```python
from build123d import *

# Parameters (mm, degrees)
F0_R     = 4
F0_R_2   = 5
F1_DEPTH = 10


with BuildPart() as f1:
    # F0 (on Front) → F1 (new body)
    with BuildSketch(Plane.XZ):
        with BuildLine():
            ThreePointArc((-128.8754135109, -25.0952865806), (-123.1602737314, -22.4552566283), (-120.8289454463, -16.6073946878))
            ThreePointArc((-120.8289454463, -16.6073946878), (-124.0394968392, -9.9536939557), (-131.2458239011, -8.326357495))
            ThreePointArc((-131.2458239011, -8.326357495), (-137.7452743032, -17.797104136), (-128.8754135109, -25.0952865806))
        make_face()
        with Locations((-129.3289454463, -16.6073946878)):
            Circle(F0_R, mode=Mode.SUBTRACT)
        with BuildLine():
            ThreePointArc((-131.2458239011, -8.326357495), (-124.0394968392, -9.9536939557), (-120.8289454463, -16.6073946878))
            ThreePointArc((-120.8289454463, -16.6073946878), (-123.1602737314, -22.4552566283), (-128.8754135109, -25.0952865806))
            add(Edge.make_bspline(
                [(27.532273017, -23.963665398), (1.5839289913, -22.6401279773), (-50.8745236246, -19.0093143919), (-102.6400941915, -24.2784335073), (-128.8754135109, -25.0952865806)],
                knots=[0.0136350591, 0.0136350591, 0.0136350591, 0.0136350591, 0.501767797, 1, 1, 1, 1], degree=3))
            ThreePointArc((27.532273017, -23.963665398), (23.6774268876, -21.8978591269), (21.6302831699, -18.0330697627))
            add(Edge.make_bspline(
                [(21.6302831699, -18.0330697627), (10.6563367579, -17.139313249), (-11.4221872367, -15.3394334373), (-44.3388932106, -14.1423054761), (-78.9588463965, -16.6641001427), (-98.3406285912, -18.1155278421)],
                knots=[0, 0, 0, 0, 0.2993707154, 0.6024154943, 0.9795111889, 0.9795111889, 0.9795111889, 0.9795111889], degree=3))
            ThreePointArc((-98.3406285912, -18.1155278421), (-100.8823299041, -17.4386421951), (-102.4541582861, -15.3296672591))
            Line((-102.4541582861, -15.3296672591), (-104.3954498587, -9.1735058104))
            ThreePointArc((-104.3954498587, -9.1735058104), (-104.0739536016, -6.0220282679), (-101.5614502719, -4.0926507615))
            add(Edge.make_bspline(
                [(83.1727162004, 25.6010051817), (69.0016849645, 24.6252928547), (38.5314258984, 22.5273363348), (-18.4508975965, 16.7813390569), (-72.1336091939, 3.3504452865), (-101.5614502719, -4.0926507615)],
                knots=[0, 0, 0, 0, 0.2783902325, 0.5985889357, 0.9821534138, 0.9821534138, 0.9821534138, 0.9821534138], degree=3))
            add(Edge.make_bspline(
                [(83.1727162004, 25.6010051817), (75.1220807527, 20.7720126759), (58.4321749927, 10.7605519796), (43.1575612073, -4.5557382523), (35.2562556315, -12.4808577154)],
                knots=[0, 0, 0, 0, 0.4823562569, 1, 1, 1, 1], degree=3))
            ThreePointArc((35.2562556315, -12.4808577154), (36.1775577554, -14.4533773309), (36.4935331712, -16.6073946878))
            ThreePointArc((36.4935331712, -16.6073946878), (36.4703721297, -17.1963591935), (36.4010320542, -17.7816860907))
            add(Edge.make_bspline(
                [(101.4293835288, 22.6709745548), (88.6185616779, 17.0455138174), (63.643555199, 8.2531548454), (45.1957048246, -8.4800882278), (36.4010320542, -17.7816860907)],
                knots=[0, 0, 0, 0, 0.5101460468, 1, 1, 1, 1], degree=3))
            ThreePointArc((101.4293835288, 22.6709745548), (94.7660609505, 27.5957675413), (99.3758214052, 34.4807920361))
            add(Edge.make_bspline(
                [(99.3758214052, 34.4807920361), (60.2046354861, 30.2118651857), (-18.683100471, 27.1404553476), (-93.822170127, 3.870933866), (-131.2458239011, -8.326357495)],
                knots=[0.0054898353, 0.0054898353, 0.0054898353, 0.0054898353, 0.5011367949, 1, 1, 1, 1], degree=3))
        make_face()
        with BuildLine():
            add(Edge.make_bspline(
                [(100.6773584463, 34.6236595183), (100.2435315443, 34.5756940781), (99.8096853764, 34.5280750966), (99.3758214052, 34.4807920361)],
                knots=[0, 0, 0, 0, 0.0054898353, 0.0054898353, 0.0054898353, 0.0054898353], degree=3))
            ThreePointArc((99.3758214052, 34.4807920361), (94.7660609505, 27.5957675413), (101.4293835288, 22.6709745548))
            ThreePointArc((101.4293835288, 22.6709745548), (105.1780334232, 24.6557980348), (106.6773584463, 28.6236595183))
            ThreePointArc((106.6773584463, 28.6236595183), (104.9199991334, 32.8663002054), (100.6773584463, 34.6236595183))
        make_face()
        with Locations((100.6773584463, 28.6236595183)):
            Circle(F0_R, mode=Mode.SUBTRACT)
        with BuildLine():
            ThreePointArc((100.6773584463, 34.6236595183), (100.0226810855, 34.5878357023), (99.3758214052, 34.4807920361))
            add(Edge.make_bspline(
                [(100.6773584463, 34.6236595183), (100.2435315443, 34.5756940781), (99.8096853764, 34.5280750966), (99.3758214052, 34.4807920361)],
                knots=[0, 0, 0, 0, 0.0054898353, 0.0054898353, 0.0054898353, 0.0054898353], degree=3))
        make_face()
        with BuildLine():
            add(Edge.make_bspline(
                [(29.7066930366, -24.0734112299), (28.9818986202, -24.0372371146), (28.2570906247, -24.000635897), (27.532273017, -23.963665398)],
                knots=[0, 0, 0, 0, 0.0136350591, 0.0136350591, 0.0136350591, 0.0136350591], degree=3))
            ThreePointArc((27.532273017, -23.963665398), (28.6154795408, -24.0978603244), (29.7066930366, -24.0734112299))
        make_face()
        with BuildLine():
            ThreePointArc((21.6302831699, -18.0330697627), (23.6774268876, -21.8978591269), (27.532273017, -23.963665398))
            add(Edge.make_bspline(
                [(29.7066930366, -24.0734112299), (28.9818986202, -24.0372371146), (28.2570906247, -24.000635897), (27.532273017, -23.963665398)],
                knots=[0, 0, 0, 0, 0.0136350591, 0.0136350591, 0.0136350591, 0.0136350591], degree=3))
            ThreePointArc((29.7066930366, -24.0734112299), (34.1299449473, -22.0724906675), (36.4010320542, -17.7816860907))
            ThreePointArc((36.4010320542, -17.7816860907), (36.4703721297, -17.1963591935), (36.4935331712, -16.6073946878))
            ThreePointArc((36.4935331712, -16.6073946878), (36.1775577554, -14.4533773309), (35.2562556315, -12.4808577154))
            ThreePointArc((35.2562556315, -12.4808577154), (26.1634174718, -9.6618605019), (21.6302831699, -18.0330697627))
        make_face()
        with Locations((28.9935331712, -16.6073946878)):
            Circle(F0_R_2, mode=Mode.SUBTRACT)
    extrude(amount=F1_DEPTH)


solid = f1.part
```
CAD build for the part. Positions are in the model's coordinates, mm. A direction names the side the tool comes from. Coordinates: 2 decimals unless noted, no trailing zeros. Return JSON: item names as keys, results as strings. Group by question number.
Q1. Drill centre lines: line 1 (X direction, y = -8, z = -13); line 2 (X direction, y = -9, z = -9); line 3 (Z direction, x = 74.5, y = -4.5). Where is each one in solid material? Low to high.
Q2. Flat gauge pins, fed straight in: pin 1 (9 mm diameter, centred on x = 100.68, z = 28.62, fed in from -Y); pin 2 (6 mm diameter, centred on x = -87, y = -6.5, fed in from -Z); pin 3 (4 mm diameter, centred on x = -98.5, y = -3, fed in from -Z); pin 4 (1.5 mm diameter, centred on x = 32.5, y = -8, fed in from -Z). Where does each tip first touch, or does it go through?
Q3. Which spindle directions (+Z, -Z, +X, -X, +Y, -Y) get a long thin tool onto all of the face, cutting with end or side? Do faces 1 (the face through (-25, -10, 18)), 2 (the face through (-104.096, -4.93, -6.062)). Say none if no direction does.
Q4. Cut at A-A, the plane y = -3. State how many separate pieces and enclosed holes the cut face has, then the cut area to 3 significant figures.
Q5. Pull direction X, two halves, no side cores. Call faces 3 (the face through (-25, 0, 18)), 4 (the face through (26.298, -4.93, -9.609)): released by +X, released by -X, zero draft, split by the parting line, or undercut.
Returned:
{
 "1": {"line 1": "x = -137.03 to -131.06, -127.6 to -103.19, 22.42 to 25.53, 32.46 to 41.05", "line 2": "x = -133.12 to -104.45, 38.73 to 45.19", "line 3": "z = 11.11 to 20.33, 25 to 32.07"},
 "2": {"pin 1": "stops at y = -10", "pin 2": "stops at z = -23.03", "pin 3": "stops at z = -23.68", "pin 4": "stops at z = -23.58"},
 "3": {"face 1": "+Z, -Z, +X, -X, -Y", "face 2": "+Y, -Y"},
 "4": {"separate pieces": "1", "enclosed holes": "4", "area": "3,350 mm2"},
 "5": {"face 3": "zero draft", "face 4": "undercut"}
}
